from build123d import *

# Parameters (mm, degrees)
SKETCH1_R           = 20
BOSS_EXTRUDE1_DEPTH = 3
SKETCH2_R           = 0.9
CUT_EXTRUDE1_DEPTH  = 3


with BuildPart() as part:
    # Sketch1 → Boss-Extrude1 (new body)
    with BuildSketch(Plane.XY):
        Circle(SKETCH1_R)
        with BuildLine():
            ThreePointArc((-6.627007241, 1.527342474), (-7.35518547, 4.260427995), (-4.622099949, 4.988606224))
            Line((-4.622099949, 4.988606224), (-1.593494167, 3.234312344))
            Line((-1.593494167, 3.234312344), (5.787770469, 13.982192711))
            ThreePointArc((5.787770469, 13.982192711), (8.037409208, 14.911223436), (9.518402344, 12.979739065))
            ThreePointArc((9.518402344, 12.979739065), (9.449886715, 12.460732201), (9.24903422, 11.977285419))
            Line((9.24903422, 11.977285419), (3.598401459, 0.226951406))
            Line((3.598401459, 0.226951406), (6.627007241, -1.527342474))
            ThreePointArc((6.627007241, -1.527342474), (7.35518547, -4.260427995), (4.622099949, -4.988606224))
            Line((4.622099949, -4.988606224), (1.593494167, -3.234312344))
            Line((1.593494167, -3.234312344), (-5.787770469, -13.982192711))
            ThreePointArc((-5.787770469, -13.982192711), (-8.52085599, -14.71037094), (-9.24903422, -11.977285419))
            Line((-9.24903422, -11.977285419), (-3.598401459, -0.226951406))
            Line((-3.598401459, -0.226951406), (-6.627007241, 1.527342474))
        make_face(mode=Mode.SUBTRACT)
    extrude(amount=BOSS_EXTRUDE1_DEPTH)

    # Sketch2 → Cut-Extrude1 (cut)
    with BuildSketch(Plane(origin=(0, 0, 0), x_dir=(-1, 0, 0), z_dir=(0, 0, -1))):
        with Locations((-2.408978249, -7.628684277)):
            Circle(SKETCH2_R)
        with Locations((-7.628684277, 2.408978249)):
            Circle(SKETCH2_R)
        with Locations((2.408978249, 7.628684277)):
            Circle(SKETCH2_R)
        with Locations((7.628684277, -2.408978249)):
            Circle(SKETCH2_R)
    extrude(amount=-CUT_EXTRUDE1_DEPTH, mode=Mode.SUBTRACT)


solid = part.part
Work out the finished part from the listing and answer in its coordinate system (mm). A direction names the side the tool comes from. Round coordinates to 2 decimals unless told otherwise and drop trailing zeros. Loops run counter-clockwise (first coordinate to the right, second up) from the corner with the lowest first, then second, coordinate; pieces in that order, holes last. Notation, with made-up numbers: (-34.5, -18) - (-24.5, -18) arc R34 cw to (-24.5, 21) - close; hole circle Ø4 at (85.5, 9). An arc over 180 degrees is marked (long way). Use one line per item in the form item = value. Start each with the question number.
(1) Find section C-C on z = 1.2. Determine the outline of the cut face in (x, y).
(2) Find section D-D on x = -16. Determine the outline of the cut face in (y, z), and give its area (3 significant figures).
(3) Flat-ended cylindrical pins translate along their axes: P1, Ø2.5, axis at x = -2.41, y = 7.63, coming from the +Z side; P2, Ø1, axis at x = 14, z = 2, coming from the -Y side; P3, Ø1.5, axis at x = -1, z = 1, coming from the -Y side; P4, Ø1.5, axis at x = 8, z = 2, coming from the +Y side. Find the tip coordinate at first contact, or state that the pin passes through.
(4) Determine the mould class of faces 3 (the face through (-3.129, 4.124, 1.479)), 4 (the face through (-6.46, -6.18, 1.48)), 5 (the face through (4.2, 0.3, 3)), 6 (the face through (-4.336, -19.524, 1.479)) for opening direction Y: +Y half, -Y half, draft (parallel to the pull), parting line (faces both ways), or undercut.
(5) Consider line 1 (Y direction, x = -7, z = 1.3) (3 decimals); line 2 (X direction, y = 4.5, z = 1.5); line 3 (X direction, y = 5, z = 2.3). Determine where each line is inside the solid, lowest interval first.
(6) Which of the six approach directions +Z, -Z, +X, -X, +Y, -Y give full straight-line access (tool end or side, diameter ignored) to faces 1 (the face through (4.2, 0.3, 0)), 2 (the face through (3.129, -4.124, 1.479))?
(7) Find section A-A on x = 2.5. Determine the outline of the cut face in (y, z).
(8) Find section B-B on y = -4.5. Determine the outline of the cut face in (x, z).
Answer list:
q1.outline = circle Ø40 at (0, 0); hole (-9.25, -11.98) arc R2 ccw to (-5.79, -13.98) - (1.59, -3.23) - (4.62, -4.99) arc R2 ccw to (6.63, -1.53) - (3.6, 0.23) - (9.25, 11.98) arc R2 ccw to (5.79, 13.98) - (-1.59, 3.23) - (-4.62, 4.99) arc R2 ccw to (-6.63, 1.53) - (-3.6, -0.23) - close; hole circle Ø1.8 at (-7.63, -2.41); hole circle Ø1.8 at (-2.41, 7.63); hole circle Ø1.8 at (2.41, -7.63); hole circle Ø1.8 at (7.63, 2.41)
q2.outline = (-12, 0) - (12, 0) - (12, 3) - (-12, 3) - close
q2.area = 72.0 mm^2
q3.P1 = 3
q3.P2 = -14.76
q3.P3 = -20
q3.P4 = 18.64
q4.face_3 = undercut
q4.face_4 = undercut
q4.face_5 = draft
q4.face_6 = parting line
q5.line_1 = -18.735 to -14.911, -7.3 to -3.053, -1.765 to 1.806, 4.71 to 18.735
q5.line_2 = -19.49 to -7.19, -3.78 to -0.72, 5.65 to 19.49
q5.line_3 = -19.36 to -6.61, -4.64 to -0.38, 5.89 to 19.36
q6.face_1 = -Z, +X, -X, +Y, -Y
q6.face_2 = +Z, -Z
q7.outline = (-19.84, 0) - (-8.52, 0) - (-8.52, 3) - (-19.84, 3) - close; (-6.73, 0) - (-3.76, 0) - (-3.76, 3) - (-6.73, 3) - close; (9.19, 0) - (19.84, 0) - (19.84, 3) - (9.19, 3) - close
q8.outline = (-19.49, 0) - (-5.65, 0) - (-5.65, 3) - (-19.49, 3) - close; (0.72, 0) - (3.78, 0) - (3.78, 3) - (0.72, 3) - close; (7.19, 0) - (19.49, 0) - (19.49, 3) - (7.19, 3) - close
